Answer from the drawing. Dimensions are ordinates in mm from the lowest x, y and z of the part. A direction names the side the tool comes from. Round coordinates to 2 decimals unless told otherwise and drop trailing zeros. Write each loop counter-clockwise with the first axis right and the second up, starting at its lowest first coordinate (ties: lowest second). Pieces come first, ordered by that corner, then holes.
1. Straight lines are drawn through the part: probe 1 along Y at (x, z) = (48, 38); probe 2 along Z at (x, y) = (50.1, 177.8) (3 decimals); probe 3 along Z at (x, y) = (48, 152). For each, find the intervals that lie inside material, in ascending order.
2. Find section D-D (x = 33.5). Write down the section's boundary in (y, z) (3 decimals).
3. Flat-ended cylindrical pins translate along their axes: pin 1 Ø3.5 at (x, z) = (19, 1.5) entering from +Y; pin 2 Ø8.5 at (y, z) = (152.4, 38.1) entering from +X; pin 3 Ø24 at (x, y) = (22.5, 103.5) entering from +Z (3 decimals); pin 4 Ø4 at (x, y) = (22.225, 76.2) entering from +Z. Find the tip coordinate at first contact, or state that the pin passes through.
4. Find section A-A (y = 38.1). Write down the section's boundary in (x, z) (3 decimals), and give its area (3 significant figures).
5. A tool of negligible diameter and unlimited length cuts with its end or side. For the marked faces 1 and 2, from which of +Z, -Z, +X, -X, +Y, -Y can it reach the whole face along a straight path? Write none if from no direction.
6. Find section C-C (y = 64.5). Write down the section's boundary in (x, z) (3 decimals).
7. Find section B-B (y = 12.7). Write down the section's boundary in (x, z) (3 decimals), and give its area (3 significant figures).
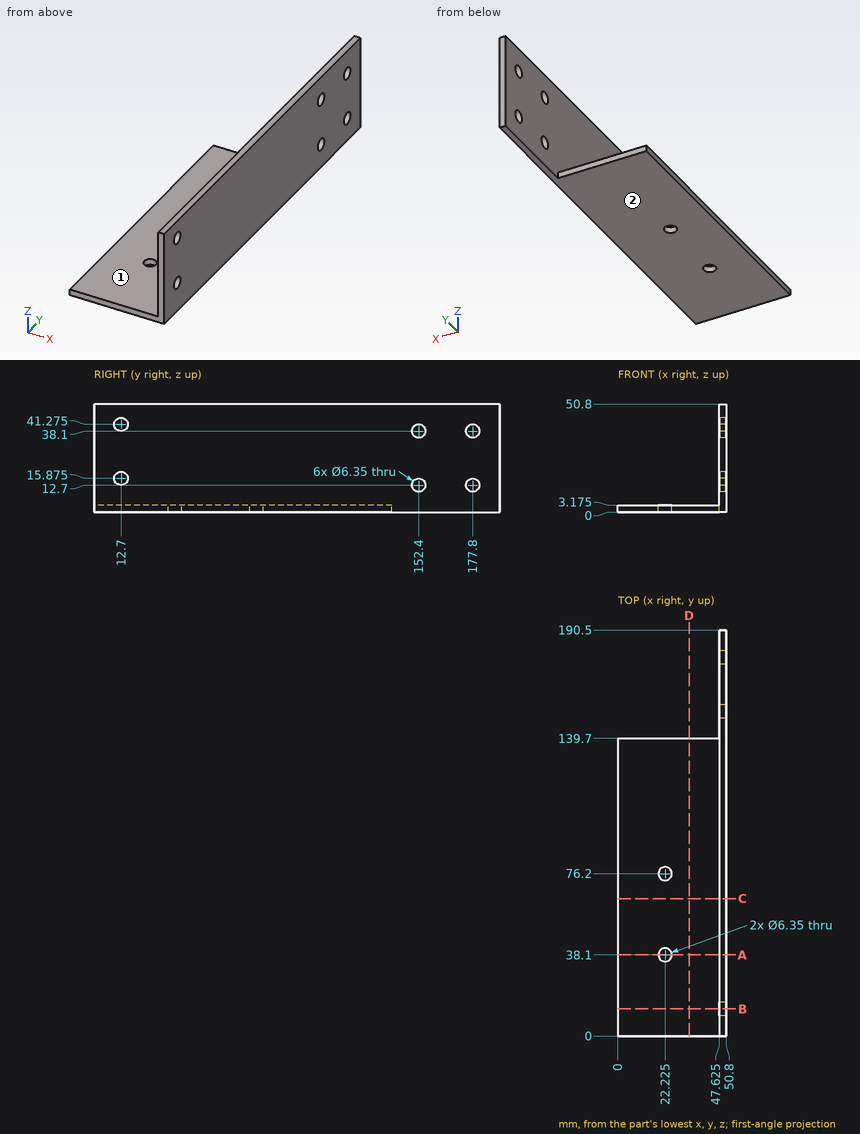
Worked answers:
1. probe 1: y = 0 to 149.23, 155.57 to 174.63, 180.97 to 190.5
1. probe 2: z = 0 to 9.525, 15.875 to 34.925, 41.275 to 50.8
1. probe 3: z = 0 to 9.55, 15.85 to 34.95, 41.25 to 50.8
2. outline: (0, 0) - (139.7, 0) - (139.7, 3.175) - (0, 3.175) - close
3. pin 1: stops at y = 139.7
3. pin 2: stops at x = 50.8
3. pin 3: stops at z = 3.175
3. pin 4: passes through
4. outline: (0, 0) - (19.05, 0) - (19.05, 3.175) - (0, 3.175) - close; (25.4, 0) - (50.8, 0) - (50.8, 50.8) - (47.625, 50.8) - (47.625, 3.175) - (25.4, 3.175) - close
4. area: 292 mm2
5. face 1: +Z, -X, +Y, -Y
5. face 2: -Z, +X, -X, +Y, -Y
6. outline: (0, 0) - (50.8, 0) - (50.8, 50.8) - (47.625, 50.8) - (47.625, 3.175) - (0, 3.175) - close
7. outline: (0, 0) - (50.8, 0) - (50.8, 12.7) - (47.625, 12.7) - (47.625, 3.175) - (0, 3.175) - close; (47.625, 19.05) - (50.8, 19.05) - (50.8, 38.1) - (47.625, 38.1) - close; (47.625, 44.45) - (50.8, 44.45) - (50.8, 50.8) - (47.625, 50.8) - close
7. area: 272 mm2
